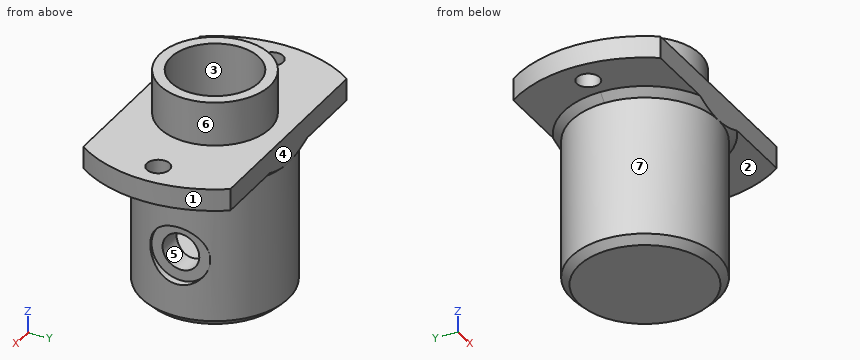
```python
from build123d import *

# Parameters (mm, degrees)
SKETCH2_R           = 10
BOSS_EXTRUDE1_DEPTH = 21
SKETCH3_R           = 1.55
BOSS_EXTRUDE3_DEPTH = 3
SKETCH4_R           = 7.5
BOSS_EXTRUDE4_DEPTH = 6
SKETCH5_R           = 6
CUT_EXTRUDE1_DEPTH  = 25
SKETCH6_R           = 4
CUT_EXTRUDE2_DEPTH  = 1
SKETCH7_R           = 2.5
CUT_EXTRUDE3_DEPTH  = 7
CHAMFER1_SIZE       = 1
CHAMFER2_SIZE       = 1


with BuildPart() as part:
    # Sketch2 → Boss-Extrude1 (new body)
    with BuildSketch(Plane.XY):
        with Locations(Location((0, 0, 0), (0, 0, 180))):
            Circle(SKETCH2_R)
    extrude(amount=BOSS_EXTRUDE1_DEPTH)

    # Sketch3 → Boss-Extrude3 (add)
    with BuildSketch(Plane.XY.offset(21)):
        with BuildLine():
            Line((14.361406616, 10), (-14.361406616, 10))
            ThreePointArc((-14.361406616, 10), (-17.5, 0), (-14.361406616, -10))
            Line((-14.361406616, -10), (14.361406616, -10))
            ThreePointArc((14.361406616, -10), (17.5, 0), (14.361406616, 10))
        make_face()
        with Locations((14, 0)):
            Circle(SKETCH3_R, mode=Mode.SUBTRACT)
        with Locations((-14, 0)):
            Circle(SKETCH3_R, mode=Mode.SUBTRACT)
    extrude(amount=BOSS_EXTRUDE3_DEPTH)

    # Sketch4 → Boss-Extrude4 (add)
    with BuildSketch(Plane.XY.offset(24)):
        Circle(SKETCH4_R)
    extrude(amount=BOSS_EXTRUDE4_DEPTH)

    # Sketch5 → Cut-Extrude1 (cut)
    with BuildSketch(Plane.XY.offset(30)):
        Circle(SKETCH5_R)
    extrude(amount=-CUT_EXTRUDE1_DEPTH, mode=Mode.SUBTRACT)

    # Sketch6 → Cut-Extrude2 (cut)
    with BuildSketch(Plane(origin=(10, 0, 0), x_dir=(0, 0, -1), z_dir=(1, 0, 0))):
        with Locations((-9.5, 0.3231801)):
            Circle(SKETCH6_R)
    extrude(amount=-CUT_EXTRUDE2_DEPTH, mode=Mode.SUBTRACT)

    # Sketch7 → Cut-Extrude3 (cut)
    with BuildSketch(Plane(origin=(9, 0, 0), x_dir=(0, 0, -1), z_dir=(1, 0, 0))):
        with Locations((-9.5, 0.3231801)):
            Circle(SKETCH7_R)
    extrude(amount=-CUT_EXTRUDE3_DEPTH, mode=Mode.SUBTRACT)

    # Chamfer1
    chamfer1_edges = [part.edges().sort_by_distance(p)[0] for p in [
        (10, 0, 0),
    ]]
    chamfer(chamfer1_edges, length=CHAMFER1_SIZE)

    # Chamfer2
    # the kernel refuses this chamfer: 1 mm, written as the material it adds along each edge
    with BuildSketch(Plane(origin=(0, 0, 21), x_dir=(-1, 0, 0), z_dir=(0, 1, 0))) as chamfer2_piece_1_section:
        Polygon((10, -CHAMFER2_SIZE), (10 + CHAMFER2_SIZE, 0), (10, 0), align=None)
    chamfer2_piece_1 = revolve(axis=Axis((0, 0, 21), (0, 0, 1)), revolution_arc=90.000000093, mode=Mode.PRIVATE)
    chamfer2_piece_1 = split(chamfer2_piece_1, bisect_by=Plane(origin=(-7.415105154, -10, 20.513457715), z_dir=(0, 1, 0)), keep=Keep.TOP, mode=Mode.PRIVATE)
    add(chamfer2_piece_1)
    with BuildSketch(Plane(origin=(0, 0, 21), x_dir=(1.6193002877922622e-09, -1.0, 0), z_dir=(-1.0, -1.6193002877922622e-09, 0))) as chamfer2_piece_2_section:
        Polygon((10, -CHAMFER2_SIZE), (10 + CHAMFER2_SIZE, 0), (10, 0), align=None)
    chamfer2_piece_2 = revolve(axis=Axis((0, 0, 21), (0, 0, 1)), revolution_arc=180.00000015, mode=Mode.PRIVATE)
    chamfer2_piece_2 = split(chamfer2_piece_2, bisect_by=Plane(origin=(10.48304434, 10, 20.516955657), z_dir=(0, -1, 0)), keep=Keep.TOP, mode=Mode.PRIVATE)
    chamfer2_piece_2 = split(chamfer2_piece_2, bisect_by=Plane(origin=(10.48304434, -10, 20.516955657), z_dir=(0, 1, 0)), keep=Keep.TOP, mode=Mode.PRIVATE)
    add(chamfer2_piece_2)
    with BuildSketch(Plane(origin=(0, 0, 21), x_dir=(-4.239322364523242e-09, 1.0, 0), z_dir=(1.0, 4.239322364523242e-09, 0))) as chamfer2_piece_3_section:
        Polygon((10, -CHAMFER2_SIZE), (10 + CHAMFER2_SIZE, 0), (10, 0), align=None)
    chamfer2_piece_3 = revolve(axis=Axis((0, 0, 21), (0, 0, 1)), revolution_arc=89.999999757, mode=Mode.PRIVATE)
    chamfer2_piece_3 = split(chamfer2_piece_3, bisect_by=Plane(origin=(-7.415105177, 10, 20.513457715), z_dir=(0, -1, 0)), keep=Keep.TOP, mode=Mode.PRIVATE)
    add(chamfer2_piece_3)


solid = part.part
```
The listing builds one solid part. Answer for the finished solid, in the listing's coordinates (mm). Face numbers are marked on the shaded views. A direction names the side the tool comes from. Coordinates: 2 decimals unless noted, no trailing zeros. Write each loop counter-clockwise with the first axis right and the second up, starting at its lowest first coordinate (ties: lowest second). Pieces come first, ordered by that corner, then holes. Notation, with made-up numbers: M 22,51 L 67,51 A22 cw 67,89 Z; hole C 82,73 d8. An arc over 180 degrees is marked long. Use a Markdown table: item, result. Add a question column.
1. Given P1, Ø11, axis at x = 0, y = 0, coming from the +Z side; P2, Ø6, axis at x = 12.5, z = 10, coming from the -Y side; P3, Ø1, axis at y = 5.5, z = 27, coming from the -X side; P4, Ø3, axis at y = -3.5, z = 11.5, coming from the -X side, each flat-ended and moving along its own axis, determine where each tip first touches the part or whether it passes through.
2. For a pull along Y with two mould halves and no side action, classify the marked faces 1, 2 and 3 as +Y half, -Y half, draft (parallel to the pull), parting line (faces both ways), or undercut.
3. Section B-B (z = 23) is taken. Give the vertices of the cut face in (x, y), plus the area to 3 significant figures.
4. Section C-C (z = 15.5) is taken. Give the vertices of the cut face in (x, y).
5. Which of the six approach directions +Z, -Z, +X, -X, +Y, -Y give full straight-line access (tool end or side, diameter ignored) to the marked faces 4, 5, 6 and 7?
6. Section D-D (y = -1) is taken. Count the separate pieces of the cut face and the enclosed holes in it, plus the area to 3 significant figures.
7. Section A-A (x = -13) is taken. Give the vertices of the cut face in (y, z).
8. Straight lines are drawn through the part: line 1 along Y through (x, z) = (14, 23); line 2 along Y through (x, z) = (0, 16); line 3 along Z through (x, y) = (12.5, 0.5). For each, find the intervals that lie inside material, in ascending order. Write a range as [from, to].
Data:
| question | item | result |
|---|---|---|
| 1 | P1 | stops at z = 5 |
| 1 | P2 | passes through |
| 1 | P3 | stops at x = -5.59 |
| 1 | P4 | stops at x = -9.8 |
| 2 | face 1 | parting line |
| 2 | face 2 | draft |
| 2 | face 3 | undercut |
| 3 | outline | M -14.36,-10 L 14.36,-10 A17.5 ccw 14.36,10 L -14.36,10 A17.5 ccw Z; hole C -14,0 d3.1; hole C 0,0 d12; hole C 14,0 d3.1 |
| 3 | area | 532 mm2 |
| 4 | outline | C 0,0 d20; hole C 0,0 d12 |
| 5 | face 4 | +Z, -Z, +X, -X, +Y |
| 5 | face 5 | +X |
| 5 | face 6 | +Z |
| 5 | face 7 | -Z |
| 6 | separate pieces | 4 |
| 6 | enclosed holes | 0 |
| 6 | area | 282 mm2 |
| 7 | outline | M -10,21 L -1.18,21 L -1.18,24 L -10,24 Z; M 1.18,21 L 10,21 L 10,24 L 1.18,24 Z |
| 8 | line 1 | y = [-10, -1.55], [1.55, 10] |
| 8 | line 2 | y = [-10, -6], [6, 10] |
| 8 | line 3 | z = [21, 24] |
